Verification items for the finished model (mm, model axes). Coordinates: 2 decimals unless noted, no trailing zeros. Order: outer loops, then holes, each group sorted by start corner. A loop starts at its lowest first (then second) coordinate and runs counter-clockwise, first axis right, second up. Notation, with made-up numbers: (-1, 46) - (31, 46) arc R20 ccw to (31, 69) - close; hole circle Ø10 at (64.25, 51.5). An arc over 180 degrees is marked (long way). Answer as CSV lines item,"result". Start each with the question number.
1. Material ranges on L1, parallel to Z at x = 87, y = -0.5; L2, parallel to Z at x = -58.5, y = -3; L3, parallel to Y at x = -59, z = 30.5, recorded low to high. Write a range as [from, to].
2. Section check B-B (z = 37.5). Record the cut outline in (x, y), and give its area (3 significant figures).
3. Go/stop test with flat-tipped pins: pin 1 (1.9 mm diameter, centred on x = -87, z = 49, fed in from -Y); pin 2 (1.8 mm diameter, centred on y = -3, z = -12, fed in from -X); pin 3 (6 mm diameter, centred on x = 68.5, z = -19.5, fed in from -Y); pin 4 (1.8 mm diameter, centred on y = -4, z = -2.5, fed in from +X). Record where each tip stops, or that it passes through.
4. Section check C-C (y = -3.8). Record the cut outline in (x, z), and give its area (3 significant figures).
5. Section check A-A (x = 73). Record the cut outline in (y, z), and give its area (3 significant figures).
from build123d import *

# Parameters (mm, degrees)
F0_W      = 180
F0_H      = 104
F0_R      = 1.6
F1_DEPTH  = 1.5748
F2_W      = 164.9
F2_H      = 100
F3_DEPTH  = 3.7
F4_W      = 156.9
F4_H      = 89
F5_DEPTH  = 0.2
F6_W      = 154.08
F6_H      = 85.92
F7_DEPTH  = 0.1
F8_R      = 0.1
F9_R      = 0.5
F10_DEPTH = 1.5758


with BuildPart() as f1:
    # F0 (on Front) → F1 (new body)
    with BuildSketch(Plane.XZ):
        Rectangle(F0_W, F0_H)
        with Locations((-87, -49)):
            Circle(F0_R, mode=Mode.SUBTRACT)
        with Locations((87, -49)):
            Circle(F0_R, mode=Mode.SUBTRACT)
        with Locations((-87, 49)):
            Circle(F0_R, mode=Mode.SUBTRACT)
        with Locations((87, 49)):
            Circle(F0_R, mode=Mode.SUBTRACT)
    extrude(amount=F1_DEPTH)

    # F2 (on face) → F3 (join)
    with BuildSketch(Plane.XZ.offset(1.5748)):
        Rectangle(F2_W, F2_H)
    extrude(amount=F3_DEPTH)

    # F4 (on face) → F5 (cut)
    with BuildSketch(Plane.XZ.offset(5.2748)):
        with Locations((-1.7, 2)):
            Rectangle(F4_W, F4_H)
    extrude(amount=-F5_DEPTH, mode=Mode.SUBTRACT)

    # F6 (on face) → F7 (join)
    with BuildSketch(Plane.XZ.offset(5.0748)):
        with Locations((-1.49, 2)):
            Rectangle(F6_W, F6_H)
    extrude(amount=F7_DEPTH)

    # F8
    f8_edges = [f1.edges().sort_by_distance(p)[0] for p in [
        (-82.45, -5.2748, 0),
        (0, -5.2748, 50),
        (0, -5.2748, -50),
        (82.45, -5.2748, 0),
    ]]
    fillet(f8_edges, radius=F8_R)

    # F9 (on face) → F10 (cut, through all)
    with BuildSketch(Plane.XZ.offset(1.5748)):
        with Locations((85.96, 13.97)):
            Circle(F9_R)
        with Locations((85.96, 8.89)):
            Circle(F9_R)
        with Locations((85.96, 11.43)):
            Circle(F9_R)
        with Locations((85.96, -19.05)):
            Circle(F9_R)
        with Locations((85.96, -16.51)):
            Circle(F9_R)
        with Locations((85.96, -13.97)):
            Circle(F9_R)
        with Locations((85.96, -11.43)):
            Circle(F9_R)
        with Locations((85.96, -8.89)):
            Circle(F9_R)
        with Locations((85.96, -6.35)):
            Circle(F9_R)
        with Locations((85.96, -3.81)):
            Circle(F9_R)
        with Locations((85.96, -1.27)):
            Circle(F9_R)
        with Locations((85.96, 3.81)):
            Circle(F9_R)
        with Locations((88.5, -16.51)):
            Circle(F9_R)
        with Locations((85.96, 6.35)):
            Circle(F9_R)
        with Locations((85.96, 16.51)):
            Circle(F9_R)
        with Locations((88.5, 19.05)):
            Circle(F9_R)
        with Locations((85.96, 19.05)):
            Circle(F9_R)
        with Locations((85.96, 21.59)):
            Circle(F9_R)
        with Locations((88.5, 21.59)):
            Circle(F9_R)
        with Locations((88.5, -19.05)):
            Circle(F9_R)
        with Locations((85.96, 24.13)):
            Circle(F9_R)
        with Locations((88.5, 13.97)):
            Circle(F9_R)
        with Locations((88.5, -8.89)):
            Circle(F9_R)
        with Locations((88.5, -1.27)):
            Circle(F9_R)
        with Locations((88.5, 16.51)):
            Circle(F9_R)
        with Locations((85.96, 1.27)):
            Circle(F9_R)
        with Locations((88.5, 24.13)):
            Circle(F9_R)
        with Locations((88.5, 6.35)):
            Circle(F9_R)
        with Locations((88.5, -6.35)):
            Circle(F9_R)
        with Locations((88.5, -21.59)):
            Circle(F9_R)
        with Locations((88.5, 1.27)):
            Circle(F9_R)
        with Locations((88.5, -13.97)):
            Circle(F9_R)
        with Locations((88.5, 8.89)):
            Circle(F9_R)
        with Locations((88.5, -3.81)):
            Circle(F9_R)
        with Locations((88.5, 3.81)):
            Circle(F9_R)
        with Locations((88.5, -11.43)):
            Circle(F9_R)
        with Locations((88.5, 11.43)):
            Circle(F9_R)
        with Locations((85.96, -24.13)):
            Circle(F9_R)
        with Locations((88.5, -24.13)):
            Circle(F9_R)
        with Locations((85.96, -21.59)):
            Circle(F9_R)
    extrude(amount=-F10_DEPTH, mode=Mode.SUBTRACT)


solid = f1.part
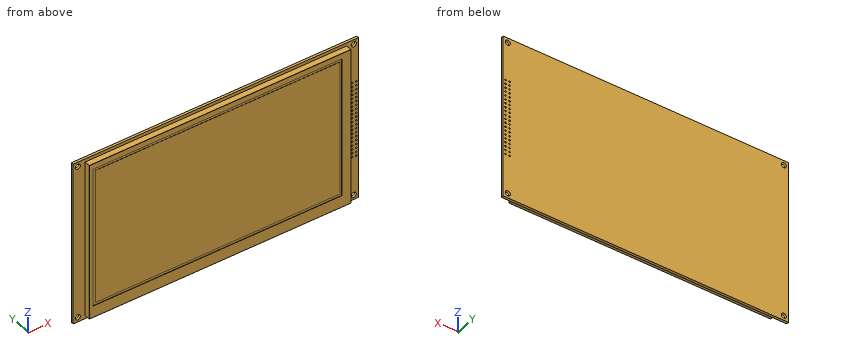
Evaluation:
1,L1,"z = [-52, -50.6], [-47.4, 47.4], [50.6, 52]"
1,L2,"z = [-50, 50]"
1,L3,"y = [-5.17, 0]"
2,outline,"(-90, -1.57) - (-82.45, -1.57) - (-82.45, -5.17) arc R0.1 ccw to (-82.35, -5.27) - (-80.15, -5.27) - (-80.15, -5.07) - (-78.53, -5.07) - (-78.53, -5.17) - (75.55, -5.17) - (75.55, -5.07) - (76.75, -5.07) - (76.75, -5.27) - (82.35, -5.27) arc R0.1 ccw to (82.45, -5.17) - (82.45, -1.57) - (90, -1.57) - (90, 0) - (-90, 0) - close"
2,area,"878 mm²"
3,pin 1,"passes through"
3,pin 2,"stops at x = -82.45"
3,pin 3,"stops at y = -5.17"
3,pin 4,"stops at x = 82.45"
4,outline,"(-82.45, -50) - (82.45, -50) - (82.45, 50) - (-82.45, 50) - close"
4,area,"16,500 mm²"
5,outline,"(-5.27, -49.9) arc R0.1 ccw to (-5.17, -50) - (-1.57, -50) - (-1.57, -52) - (0, -52) - (0, 52) - (-1.57, 52) - (-1.57, 50) - (-5.17, 50) arc R0.1 ccw to (-5.27, 49.9) - (-5.27, 46.5) - (-5.07, 46.5) - (-5.07, 44.96) - (-5.17, 44.96) - (-5.17, -40.96) - (-5.07, -40.96) - (-5.07, -42.5) - (-5.27, -42.5) - close"
5,area,"525 mm²"
